Verification items for the finished model (mm, model axes). Face numbers are marked on the shaded views. A direction names the side the tool comes from. Give positions to 0.01 mm unless a question says otherwise; leave off trailing zeros. Loops run counter-clockwise (first coordinate to the right, second up) from the corner with the lowest first, then second, coordinate; pieces in that order, holes last. Notation, with made-up numbers: (77.25, -25) -> (127.25, -25) arc R12 ccw to (127.25, -4) -> close; hole circle Ø3 at (49, -32). An arc over 180 degrees is marked (long way). Answer in a Markdown table with one row per item. Add a question column.
Q1. Section check B-B on z = -15.75. Give the number of separate pieces and of enclosed holes in the cut face, and give its area (4 significant figures).
Q2. Material ranges on probe 1 along Y at (x, z) = (0, -17); probe 2 along Y at (x, z) = (21.5, -15.5); probe 3 along Z at (x, y) = (12.5, -6.5), recorded low to high.
Q3. Release check for a two-part mould opening along X. For the marked faces 3 and 4 record: pulls with the +X half, pulls with the -X half, needs draft (parallel to the pull), parting line crosses it, or undercut.
Q4. Gauge pin test, flat ends, axial feed: P1, Ø3.5, axis at x = 5.5, y = -13, coming from the +Z side; P2, Ø1.6, axis at x = 53, y = -12, coming from the +Z side; P3, Ø11.5, axis at x = 22.5, z = -16.5, coming from the +Y side; P4, Ø7, axis at x = 46.5, z = -11, coming from the -Y side. Record the tip position at first contact, or that the pin passes through.
Q5. Set-up check for the marked faces 1 and 2: record each of +Z, -Z, +X, -X, +Y, -Y from which the full face is reachable in a straight line by a thin tool's end or side.
Q6. Section check A-A on x = 1. Enter the section's corners in (y, z).
Autodesk Inventor part; units mm, degrees
ref_plane "YZ Plane" through (0, 0, 0) normal (1, 0, 0) x (0, 1, 0)
ref_plane "XZ Plane" through (0, 0, 0) normal (0, 1, 0) x (-1, 0, 0)
ref_plane "XY Plane" through (0, 0, 0) normal (0, 0, 1) x (1, 0, 0)
sketch "スケッチ1" plane through (0, 0, 0) normal (0, 0, 1) x (1, 0, 0)
  line L0 (-11.5, 13) -> (-11.5, -13)
  line L1 (11.5, 13) -> (-11.5, 13)
  line L2 (11.5, -13) -> (11.5, 13)
  line L3 (-11.5, -13) -> (11.5, -13)
  line L4 (11.5, 13) -> (63.5, 13)
  line L5 (63.5, 13) -> (63.5, -13)
  line L6 (63.5, -13) -> (11.5, -13)
  line L7 (11.5, -13) -> (11.5, 13)
  line L8 (37.5, 13) -> (37.5, -13)
  line L9 (11.5, 13) -> (37.5, -13)
  line L10 (37.5, 13) -> (11.5, -13)
  line L11 (63.5, 13) -> (37.5, -13)
  line L12 (37.5, 13) -> (63.5, -13)
  line L13 (13, -11.5) -> (62, -11.5)
  line L14 (62, 11.5) -> (13, 11.5)
  line L15 (13, -11.5) -> (13, 11.5)
  line L16 (62, -11.5) -> (62, 11.5)
  line L17 (13, -13) -> (37.5, 11.5)
  line L18 (11.5, -11.5) -> (36, 13)
  line L19 (37.5, -11.5) -> (14.5, 11.5)
  line L20 (13, 10) -> (36, -13)
  line L21 (37.5, -11.5) -> (60.5, 11.5)
  line L22 (62, 10) -> (39, -13)
  line L23 (38.0069, 10.9931) -> (60.5, -11.5)
  line L24 (62, -10) -> (39, 13)
  line L25 (37.5, 11.5) -> (60.5, -11.5)
  point P0 (0, 0)
  point P1 (49, 0)
  point P2 (26, 0)
  point P3 (13, -10)
  point P4 (23, 0)
  point P5 (34.5, 11.5)
  point P6 (24.5, 1.5)
  point P7 (14.5, -11.5)
  point P8 (24.5, -1.5)
  point P9 (34.5, -11.5)
  point P10 (40.5, -11.5)
  point P11 (50.5, -1.5)
  point P12 (52, 0)
  point P13 (40.5, 11.5)
  point P14 (50.5, 1.5)
  dimension "d0" = 52
  dimension "d1" = 26
  dimension "d2" = 1.5
extrude "押し出し1" add sketch "スケッチ1" against normal blind 1.5 contours L9 L15 L18 L2 | L4 L18 L14 L9 | L10 L13 L17 L6 | L2 L18 L15 L10 | L4 L10 L14 L18 | L14 L19 L18 L9 | L9 L18 L20 L15 | L17 L13 L20 L6 | L15 L18 L20 L10 | L10 L20 L17 L13 | L12 L14 L8 | L8 L14 L10 | L4 L24 L14 L12 | L14 L10 L19 L18 | L18 L19 L10 L9 | L9 L10 L20 L18 | L20 L13 L9 L6 | L10 L9 L17 L20 | L4 L11 L14 L24 | L17 L19 L10 L14 | L14 L12 L21 L23 L25 | L14 L24 L21 L12 | L10 L19 L17 L9 | L11 L13 L22 L6 | L9 L13 L8 | L8 L13 L11 | L20 L17 L9 L13 | L5 L12 L16 L11 | L21 L23 L11 L13 | L13 L9 L17 L19 | L21 L24 L11 L12 | L12 L11 L23 L21 | L22 L13 L12 L6 | L11 L23 L22 L13 | L16 L22 L24 L11 | L11 L24 L21 L14 | L12 L22 L23 L11 | L11 L24 L22 L12 | L13 L23 L22 L12 | L12 L22 L24 L16
sketch "スケッチ5" plane through (11.5, 13, 0) normal (0, 1, 0) x (1, 0, 0)
  line L0 (-7, 32) -> (0, 32)
  line L1 (0, 32) -> (0, 0)
  line L2 (0, 0) -> (-23, 0)
  line L3 (52, 0) -> (0, 0)
  line L4 (52, 0) -> (52, 26)
  line L5 (52, 26) -> (0, 26)
  line L6 (1.5, 26) -> (1.5, 0)
  line L7 (0, 24.5) -> (52, 24.5)
  line L8 (50.5, 26) -> (50.5, 0)
  line L9 (0, 1.5) -> (52, 1.5)
  line L10 (26, 1.5) -> (26, 26)
  line L11 (0, 26) -> (26, 0)
  line L12 (52, 26) -> (26, 0)
  line L13 (1.5, 26) -> (26, 1.5)
  line L14 (26, 1.5) -> (50.5, 26)
  line L15 (52, 24.5) -> (27.5, 0)
  line L16 (24.5, 0) -> (0, 24.5)
  line L17 (0, 0) -> (26, 26)
  line L18 (26, 26) -> (52, 0)
  line L19 (52, 1.5) -> (27.5, 26)
  line L20 (26, 24.5) -> (50.5, 0)
  line L21 (26, 24.5) -> (1.5, 0)
  line L22 (0, 1.5) -> (24.5, 26)
  point P0 (-11.5, 0)
  point P1 (49, 1.5)
  point P2 (29, 1.5)
  point P3 (39, 11.5)
  point P4 (14.5, 13)
  point P5 (37.5, 13)
  point P6 (3, 1.5)
  point P7 (13, 11.5)
  point P8 (23, 1.5)
  point P9 (50.5, 3)
  point P10 (40.5, 13)
  point P11 (50.5, 23)
  point P12 (29, 24.5)
  point P13 (49, 24.5)
  point P14 (39, 14.5)
  point P15 (1.5, 3)
  point P16 (1.5, 23)
  point P17 (11.5, 13)
  point P18 (3, 24.5)
  point P19 (23, 24.5)
  point P20 (13, 14.5)
  dimension "d7" = 26
  dimension "d8" = 1.5
  dimension "d9" = 1.5
  dimension "d10" = 1.5
extrude "押し出し2" add sketch "スケッチ5" against normal blind 1.5 contours L11 L7 L1 | L5 L6 L11 | L16 L6 L22 L1 | L7 L6 L16 | L13 L7 L6 | L5 L22 L7 L13 | L11 L22 L16 L6 | L7 L13 L22 L11 | L9 L17 L1 | L22 L6 L9 | L5 L17 L7 L22 | L22 L13 L17 L11 | L11 L17 L16 L22 | L17 L6 L3 | L9 L21 L6 | L17 L16 L21 L9 | L6 L22 L16 L17 | L18 L7 L10 | L10 L7 L17 | L5 L19 L7 L18 | L7 L17 L13 L22 | L17 L13 L21 L11 | L11 L21 L16 L17 | L21 L9 L16 L3 | L5 L14 L7 L19 | L21 L13 L17 L7 | L7 L18 L14 L20 | L7 L19 L14 L18 | L21 L13 L9 L11 | L11 L9 L16 L21 | L16 L9 L11 L3 | L5 L12 L8 | L8 L7 L14 | L9 L12 L11 | L14 L20 L12 L9 | L14 L18 L12 L20 | L14 L19 L12 L18 | L12 L9 L15 L3 | L4 L7 L12 | L12 L19 L14 L7 | L7 L15 L8 | L8 L15 L19 L12 | L12 L20 L15 L9 | L12 L18 L15 L20 | L12 L19 L15 L18 | L15 L9 L20 L3 | L4 L19 L8 L15 | L15 L18 L9 L20 | L15 L19 L8 L18 | L8 L18 L3 | L20 L9 L8 | L4 L18 L9 | L9 L8 L19
sketch "スケッチ6" plane through (11.5, -13, 0) normal (0, -1, 0) x (1, 0, 0)
  line L0 (1.5, -3) -> (11.5, -13)
  line L1 (13, -11.5) -> (3, -1.5)
  line L2 (52, -1.5) -> (0, -1.5)
  line L3 (0, 0) -> (52, 0)
  line L4 (0, -32) -> (0, 0)
  line L5 (1.5, -23) -> (1.5, -3)
  line L6 (11.5, -13) -> (1.5, -23)
  line L7 (3, -24.5) -> (13, -14.5)
  line L8 (23, -24.5) -> (3, -24.5)
  line L9 (0, -26) -> (52, -26)
  line L10 (13, -14.5) -> (23, -24.5)
  line L11 (26, -24.5) -> (14.5, -13)
  line L12 (14.5, -13) -> (26, -1.5)
  line L13 (23, -1.5) -> (13, -11.5)
  line L14 (39, -11.5) -> (29, -1.5)
  line L15 (26, -1.5) -> (37.5, -13)
  line L16 (29, -24.5) -> (39, -14.5)
  line L17 (37.5, -13) -> (26, -24.5)
  line L18 (49, -24.5) -> (29, -24.5)
  line L19 (39, -14.5) -> (49, -24.5)
  line L20 (50.5, -23) -> (40.5, -13)
  line L21 (50.5, -3) -> (50.5, -23)
  line L22 (52, -26) -> (52, -1.5)
  line L23 (40.5, -13) -> (50.5, -3)
  line L24 (49, -1.5) -> (39, -11.5)
  line L25 (52, 0) -> (52, -1.5)
  point P0 (-11.5, 0)
extrude "押し出し3" add sketch "スケッチ6" against normal blind 1.5 contours L13 L2 L14 L24 L22 L9 L4 L1 | L2 L4 L3 L25
sketch "スケッチ7" plane through (63.5, 13, -26) normal (0, 0, -1) x (-1, 0, 0)
  line L0 (50.5, -3) -> (50.5, -23)
  line L1 (40.5, -13) -> (50.5, -3)
  line L2 (49, -1.5) -> (39, -11.5)
  line L3 (52, -1.5) -> (0, -1.5)
  line L4 (39, -11.5) -> (29, -1.5)
  line L5 (26, -1.5) -> (37.5, -13)
  line L6 (37.5, -13) -> (26, -24.5)
  line L7 (29, -24.5) -> (39, -14.5)
  line L8 (39, -14.5) -> (49, -24.5)
  line L9 (0, -24.5) -> (52, -24.5)
  line L10 (52, 0) -> (52, -7)
  line L11 (52, -19) -> (52, -7)
  line L12 (52, -19) -> (52, -26)
  line L13 (52, -26) -> (0, -26)
  line L14 (0, 0) -> (52, 0)
  line L15 (14.5, -13) -> (26, -1.5)
  line L16 (26, -24.5) -> (14.5, -13)
  line L17 (13, -14.5) -> (23, -24.5)
  line L18 (3, -24.5) -> (13, -14.5)
  line L19 (11.5, -13) -> (1.5, -23)
  line L20 (1.5, -3) -> (11.5, -13)
  line L21 (13, -11.5) -> (3, -1.5)
  line L22 (23, -1.5) -> (13, -11.5)
  line L23 (1.5, -23) -> (1.5, -3)
  line L24 (0, -1.5) -> (0, -24.5)
  line L25 (0, 0) -> (0, -1.5)
  line L26 (0, -26) -> (0, -24.5)
  line L27 (50.5, -23) -> (40.5, -13)
  point P0 (63.5, -13)
extrude "押し出し4" add sketch "スケッチ7" against normal blind 1.5 contours L3 L10 L11 L12 L9 L8 L7 L6 L5 L4 L2 | L3 L25 L14 L10 | L15 L16 L9 L17 L18 L24 L3 L21 L22 | L12 L13 L26 L9
sketch "スケッチ8" plane through (0, 0, 0) normal (0, 0, 1) x (1, 0, 0)
  line L0 (11.5, 13) -> (-11.5, 13)
  line L1 (11.5, -13) -> (11.5, 13)
  line L2 (11.5, 13) -> (-11.5, 13)
  line L3 (-11.5, 13) -> (-11.5, -13)
  line L4 (-11.5, -13) -> (11.5, -13)
  circle A0 centre (0, 0) radius 5
  line L5 (40.5, -11.5) -> (50.5, -1.5)
  line L6 (50.5, -1.5) -> (60.5, -11.5)
  line L7 (60.5, -11.5) -> (40.5, -11.5)
  line L8 (63.5, -13) -> (63.5, 13)
  line L9 (63.5, 13) -> (11.5, 13)
  line L10 (11.5, 13) -> (11.5, -13)
  line L11 (11.5, -13) -> (63.5, -13)
  line L12 (37.5, -11.5) -> (26, 0)
  line L13 (26, 0) -> (37.5, 11.5)
  line L14 (37.5, 11.5) -> (49, 0)
  line L15 (49, 0) -> (37.5, -11.5)
  line L16 (34.5, -11.5) -> (14.5, -11.5)
  line L17 (14.5, -11.5) -> (24.5, -1.5)
  line L18 (24.5, -1.5) -> (34.5, -11.5)
  line L19 (34.5, 11.5) -> (24.5, 1.5)
  line L20 (24.5, 1.5) -> (14.5, 11.5)
  line L21 (14.5, 11.5) -> (34.5, 11.5)
  line L22 (40.5, 11.5) -> (60.5, 11.5)
  line L23 (60.5, 11.5) -> (50.5, 1.5)
  line L24 (50.5, 1.5) -> (40.5, 11.5)
  line L25 (13, -10) -> (13, 10)
  line L26 (13, 10) -> (23, 0)
  line L27 (23, 0) -> (13, -10)
  line L28 (52, 0) -> (62, 10)
  line L29 (62, 10) -> (62, -10)
  line L30 (62, -10) -> (52, 0)
  line L31 (13, 10) -> (13, 14.5)
  line L32 (4.5, 13) -> (4.5, 11.5)
  line L33 (4.5, 11.5) -> (10, 11.5)
  line L34 (10, 11.5) -> (10, 6)
  line L35 (10, 6) -> (11.5, 6)
  line L36 (-4.5, 11.5) -> (-4.5, 13)
  line L37 (-10, 11.5) -> (-4.5, 11.5)
  line L38 (-10, 6) -> (-10, 11.5)
  line L39 (-11.5, 6) -> (-10, 6)
  line L40 (13, 14.5) -> (-4.5, 14.5)
  line L41 (-4.5, 14.5) -> (-4.5, 11.5)
  line L42 (-4.5, 11.5) -> (4.5, 11.5)
  line L43 (4.5, 13) -> (11.5, 13)
  line L44 (-4.5, -13) -> (-4.5, -11.5)
  line L45 (-4.5, -11.5) -> (-10, -11.5)
  line L46 (-10, -11.5) -> (-10, -6)
  line L47 (-10, -6) -> (-11.5, -6)
  line L48 (4.5, -11.5) -> (4.5, -13)
  line L49 (10, -11.5) -> (4.5, -11.5)
  line L50 (10, -6) -> (10, -11.5)
  line L51 (11.5, -6) -> (10, -6)
  line L52 (13, -13) -> (23, -13)
  line L53 (13, -13) -> (13, -14.5)
  line L54 (13, -14.5) -> (-4.5, -14.5)
  line L55 (-4.5, -14.5) -> (-4.5, -11.5)
  line L56 (-4.5, -11.5) -> (4.5, -11.5)
  line L57 (4.5, -13) -> (4.5, -11.5)
  line L58 (4.5, -13) -> (11.5, -13)
  point P0 (13, 12.25)
  point P1 (13, 13)
  dimension "d17" = 4.5
  dimension "d19" = 1.5
extrude "押し出し5" add sketch "スケッチ8" against normal blind 24.5 from surface at -1.5 contours L0 L41 L40 L31 L9 | L32 L42 L36 L0 | L11 L53 L54 L55 L4 | L4 L44 L56 L48
properties part number "足フレーム"
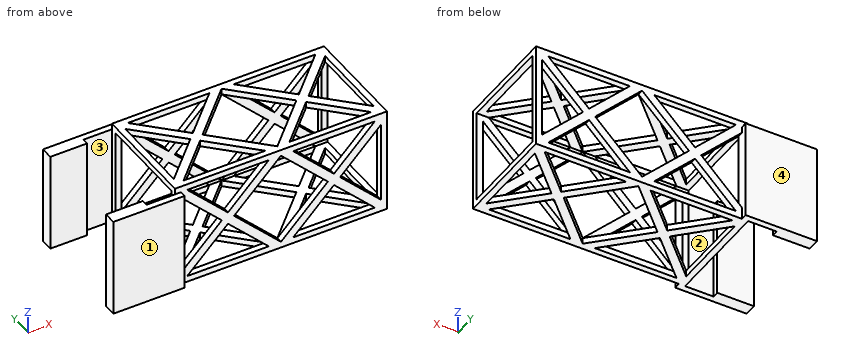
Taken from the geometry:
| question | item | result |
|---|---|---|
| 1 | separate pieces | 12 |
| 1 | enclosed holes | 0 |
| 1 | area | 124.5 mm² |
| 2 | probe 1 | y = -14.5 to -11.5, 11.5 to 14.5 |
| 2 | probe 2 | y = -13 to -11.5, 11.5 to 13 |
| 2 | probe 3 | z = -26 to -24.5, -1.5 to 0 |
| 3 | face 3 | undercut |
| 3 | face 4 | needs draft |
| 4 | P1 | stops at z = -1.5 |
| 4 | P2 | stops at z = 0 |
| 4 | P3 | stops at y = 13 |
| 4 | P4 | stops at y = -13 |
| 5 | face 1 | +Z, -Z, +X, -X, -Y |
| 5 | face 2 | +Z, -Z |
| 6 | outline | (-14.5, -26) -> (-11.5, -26) -> (-11.5, -1.5) -> (-14.5, -1.5) -> close; (11.5, -26) -> (14.5, -26) -> (14.5, -1.5) -> (11.5, -1.5) -> close |
